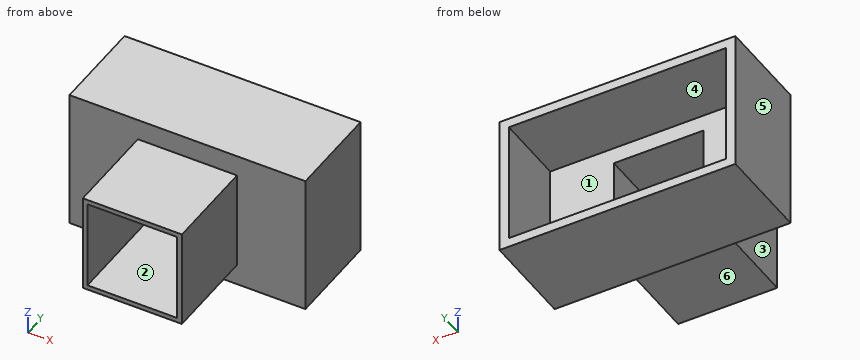
from build123d import *

# Parameters (mm, degrees)
SKETCH2_W           = 21
SKETCH2_H           = 21
BOSS_EXTRUDE1_DEPTH = 20
SKETCH3_W           = 19
SKETCH3_H           = 19
CUT_EXTRUDE1_DEPTH  = 21
SKETCH4_W           = 50
SKETCH4_H           = 30
BOSS_EXTRUDE2_DEPTH = 20
SKETCH5_W           = 46
SKETCH5_H           = 26
CUT_EXTRUDE2_DEPTH  = 15
SKETCH6_W           = 19
SKETCH6_H           = 19
CUT_EXTRUDE3_DEPTH  = 15


with BuildPart() as part:
    # Sketch2 → Boss-Extrude1 (new body)
    with BuildSketch(Plane(origin=(0, 0, 0), x_dir=(1, 0, 0), z_dir=(0, 1, 0))):
        with Locations((0.794117647, -2.823529412)):
            Rectangle(SKETCH2_W, SKETCH2_H)
    extrude(amount=BOSS_EXTRUDE1_DEPTH)

    # Sketch3 → Cut-Extrude1 (cut, through all)
    with BuildSketch(Plane(origin=(0, 20, 0), x_dir=(1, 0, 0), z_dir=(0, 1, 0))):
        with Locations((0.794117647, -2.823529412)):
            Rectangle(SKETCH3_W, SKETCH3_H)
    extrude(amount=-CUT_EXTRUDE1_DEPTH, mode=Mode.SUBTRACT)

    # Sketch4 → Boss-Extrude2 (add)
    with BuildSketch(Plane(origin=(0, 20, 0), x_dir=(1, 0, 0), z_dir=(0, 1, 0))):
        with Locations((0.794117647, -2.823529412)):
            Rectangle(SKETCH4_W, SKETCH4_H)
    extrude(amount=BOSS_EXTRUDE2_DEPTH)

    # Sketch5 → Cut-Extrude2 (cut)
    with BuildSketch(Plane(origin=(0, 40, 0), x_dir=(1, 0, 0), z_dir=(0, 1, 0))):
        with Locations((0.794117647, -2.823529412)):
            Rectangle(SKETCH5_W, SKETCH5_H)
    extrude(amount=-CUT_EXTRUDE2_DEPTH, mode=Mode.SUBTRACT)

    # Sketch6 → Cut-Extrude3 (cut)
    with BuildSketch(Plane.XZ.offset(-20)):
        with Locations((0.794117647, 2.823529412)):
            Rectangle(SKETCH6_W, SKETCH6_H)
    extrude(amount=-CUT_EXTRUDE3_DEPTH, mode=Mode.SUBTRACT)


solid = part.part
Build history of the part. All positions in model axes, mm. Face numbers are marked on the shaded views. A direction names the side the tool comes from. Give positions to 0.01 mm unless a question says otherwise; leave off trailing zeros. Loops run counter-clockwise (first coordinate to the right, second up) from the corner with the lowest first, then second, coordinate; pieces in that order, holes last. Notation, with made-up numbers: (23, 18.5) - (65, 18.5) arc R9 cw to (65, 25.5) - close; hole circle Ø9 at (41, 26.25). An arc over 180 degrees is marked (long way). Write item = value, one per line. Start each with the question number.
1) Band-saw the part on D-D on x = 17.5. Give the cut face in (y, z), plus the area to 3 significant figures.
2) Pull direction Z, two halves, no side cores. Call the marked faces 4, 5 and 6: +Z half, -Z half, draft (parallel to the pull), parting line (faces both ways), or undercut.
3) Probe probe 1 along Z at (x, y) = (2, 10.5); probe 2 along X at (y, z) = (12.5, 7); probe 3 along Z at (x, y) = (-18.5, 37). List the from-to ranges inside material, lowest first. Write a range as from..to.
4) Band-saw the part on B-B on y = 23.5. Give the cut face in (x, z).
5) Band-saw the part on A-A on z = -2.75. Give the cut face in (x, y), plus the area to 3 significant figures.
6) Tool access for the marked faces 1, 2 and 3: list every direction of +Z, -Z, +X, -X, +Y, -Y with a clear straight run to the whole face (end or side of a thin tool).
7) Drop flat-ended pins along their axis: pin 1 Ø5.5 at (x, y) = (1, 12) entering from +Z; pin 2 Ø15 at (y, z) = (6.5, 7) entering from +X; pin 3 Ø6 at (x, y) = (-0.5, 11.5) entering from -Z. Give the stop position or say it passes through.
8) Band-saw the part on C-C on x = 8. Give the cut face in (y, z), plus the area to 3 significant figures.
Final values:
q1.outline = (20, -12.18) - (40, -12.18) - (40, -10.18) - (25, -10.18) - (25, 15.82) - (40, 15.82) - (40, 17.82) - (20, 17.82) - close
q1.area = 210 mm²
q2.face_4 = undercut
q2.face_5 = draft
q2.face_6 = -Z half
q3.probe_1 = -7.68..-6.68, 12.32..13.32
q3.probe_2 = -9.71..-8.71, 10.29..11.29
q3.probe_3 = -12.18..-10.18, 15.82..17.82
q4.outline = (-24.21, -12.18) - (25.79, -12.18) - (25.79, 17.82) - (-24.21, 17.82) - close; hole (-8.71, -6.68) - (10.29, -6.68) - (10.29, 12.32) - (-8.71, 12.32) - close
q5.outline = (-24.21, 20) - (-9.71, 20) - (-9.71, 0) - (-8.71, 0) - (-8.71, 25) - (-22.21, 25) - (-22.21, 40) - (-24.21, 40) - close; (10.29, 0) - (11.29, 0) - (11.29, 20) - (25.79, 20) - (25.79, 40) - (23.79, 40) - (23.79, 25) - (10.29, 25) - close
q5.area = 255 mm²
q6.face_1 = +Y
q6.face_2 = +Y, -Y
q6.face_3 = +Z, -Z, -X, -Y
q7.pin_1 = 13.32
q7.pin_2 = 11.29
q7.pin_3 = -7.68
q8.outline = (0, -7.68) - (20, -7.68) - (20, -12.18) - (40, -12.18) - (40, -10.18) - (25, -10.18) - (25, -6.68) - (0, -6.68) - close; (0, 12.32) - (25, 12.32) - (25, 15.82) - (40, 15.82) - (40, 17.82) - (20, 17.82) - (20, 13.32) - (0, 13.32) - close
q8.area = 155 mm²
